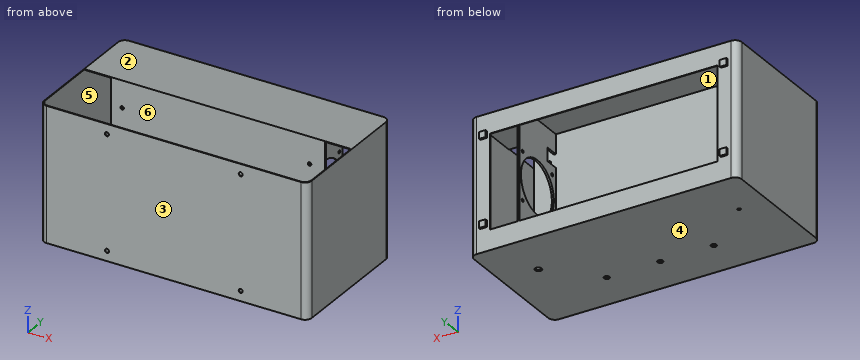
```python
from build123d import *

# Parameters (mm, degrees)
SKETCH1_W                 = 400
SKETCH1_H                 = 200
KHUNG_TRONG_DEPTH         = 100
SKETCH2_W                 = 398
SKETCH2_H                 = 198
DO_DAY_1MM_DEPTH          = 198
FILLET_10MM_4_GOC_R       = 10
SKETCH3_W                 = 320
SKETCH3_H                 = 3
TRAN_GIA_DEPTH            = 198
SKETCH5_W                 = 3
SKETCH5_H                 = 198
GIA_DO_QUAT_DEPTH         = 89
SKETCH6_R                 = 40
LO_DAT_QUAT_DEPTH         = 3
SKETCH7_R                 = 2.3
CO_DINH_QUAT_DEPTH        = 3
SKETCH9_W                 = 20
SKETCH9_H                 = 20
LO_THONG_CHO_DEN_DEPTH    = 3
SKETCH10_R                = 2.6
GIA_DO_DEN_DEPTH          = 3
DAY_NGUON_DEN_QUAT_REACH  = 491.085
SKETCH12_R                = 5
DAY_NGUON_DEN_REACH       = 491.085
SKETCH13_R                = 2.5
F_2_THANH_RAY_TANG1_REACH = 459.822
SKETCH14_R                = 3
GAN_CAM_BIEN_REACH        = 491.085
SKETCH15_R                = 4.1
SKETCH16_W                = 340
SKETCH16_H                = 140
NAP_THAM_DEPTH            = 1
SKETCH18_W                = 399
SKETCH18_H                = 1
CHE_TRAN_DEPTH            = 93
FILLET4_R                 = 10
SKETCH19_W                = 10
SKETCH19_H                = 10
CHOT_CO_DINH_DEPTH        = 3


with BuildPart() as part:
    # Sketch1 → khung_trong (new, symmetric)
    with BuildSketch(Plane.XY):
        with Locations((200, 100)):
            Rectangle(SKETCH1_W, SKETCH1_H)
    extrude(amount=KHUNG_TRONG_DEPTH, both=True)

    # Sketch2 → do_day_1mm (cut)
    with BuildSketch(Plane.XY.offset(100)):
        with Locations((200, 100)):
            Rectangle(SKETCH2_W, SKETCH2_H)
    extrude(amount=-DO_DAY_1MM_DEPTH, mode=Mode.SUBTRACT)

    # Fillet_10mm_4_goc
    fillet_10mm_4_goc_edges = [part.edges().sort_by_distance(p)[0] for p in [
        (1, 1, 1),
        (1, 199, 1),
        (399, 199, 1),
        (399, 1, 1),
        (0, 200, 0),
        (400, 200, 0),
        (400, 0, 0),
        (0, 0, 0),
    ]]
    fillet(fillet_10mm_4_goc_edges, radius=FILLET_10MM_4_GOC_R)

    # Sketch3 → tran_gia (add)
    with BuildSketch(Plane.XY.offset(-98)):
        with Locations((200, 108.5)):
            Rectangle(SKETCH3_W, SKETCH3_H)
    extrude(amount=TRAN_GIA_DEPTH)

    # Sketch5 → gia_do_quat (add)
    with BuildSketch(Plane(origin=(0, 110, 0), x_dir=(1, 0, 0), z_dir=(0, 1, 0))):
        with Locations((328.5, -1)):
            Rectangle(SKETCH5_W, SKETCH5_H)
    extrude(amount=GIA_DO_QUAT_DEPTH)

    # Sketch6 → lo_dat_quat (cut)
    with BuildSketch(Plane.ZY.offset(-327)):
        with Locations((0, 155)):
            Circle(SKETCH6_R)
    extrude(amount=-LO_DAT_QUAT_DEPTH, mode=Mode.SUBTRACT)

    # Sketch7 → co_dinh_quat (cut)
    with BuildSketch(Plane.ZY.offset(-327)):
        with Locations((-35.75, 190.75)):
            Circle(SKETCH7_R)
        with Locations((35.75, 190.75)):
            Circle(SKETCH7_R)
        with Locations((35.75, 119.25)):
            Circle(SKETCH7_R)
        with Locations((-35.75, 119.25)):
            Circle(SKETCH7_R)
    extrude(amount=-CO_DINH_QUAT_DEPTH, mode=Mode.SUBTRACT)

    # Sketch9 → lo_thong_cho _den (cut)
    with BuildSketch(Plane.ZY.offset(-327)):
        with Locations((-58, 120)):
            Rectangle(SKETCH9_W, SKETCH9_H)
        with Locations((60, 120)):
            Rectangle(SKETCH9_W, SKETCH9_H)
    extrude(amount=-LO_THONG_CHO_DEN_DEPTH, mode=Mode.SUBTRACT)

    # Sketch10 → gia_do_den (cut)
    with BuildSketch(Plane(origin=(0, 110, 0), x_dir=(1, 0, 0), z_dir=(0, 1, 0))):
        with Locations(Location((337, 58, 0), (0, 0, 270))):
            Circle(SKETCH10_R)
        with Locations(Location((337, -60, 0), (0, 0, 270))):
            Circle(SKETCH10_R)
        with Locations(Location((57, 58, 0), (0, 0, 270))):
            Circle(SKETCH10_R)
        with Locations(Location((57, -60, 0), (0, 0, 270))):
            Circle(SKETCH10_R)
    extrude(amount=-GIA_DO_DEN_DEPTH, mode=Mode.SUBTRACT)

    # Sketch12 → day_nguon_den_quat (cut, up to next)
    with BuildSketch(Plane.XY.offset(-98), mode=Mode.PRIVATE) as day_nguon_den_quat_sk1:
        with Locations((344, 125)):
            Circle(SKETCH12_R)
    day_nguon_den_quat_tool1 = extrude(day_nguon_den_quat_sk1.sketch, amount=-DAY_NGUON_DEN_QUAT_REACH, mode=Mode.PRIVATE) & part.part
    add(day_nguon_den_quat_tool1.solids().sort_by_distance((344, 125, -98))[0], mode=Mode.SUBTRACT)

    # Sketch13 → day_nguon_den (cut, up to next)
    with BuildSketch(Plane.XY.offset(-98), mode=Mode.PRIVATE) as day_nguon_den_sk1:
        with Locations((44, 125)):
            Circle(SKETCH13_R)
    day_nguon_den_tool1 = extrude(day_nguon_den_sk1.sketch, amount=-DAY_NGUON_DEN_REACH, mode=Mode.PRIVATE) & part.part
    add(day_nguon_den_tool1.solids().sort_by_distance((44, 125, -98))[0], mode=Mode.SUBTRACT)

    # Sketch14 → 2_thanh_ray_tang1 (cut, up to next)
    with BuildSketch(Plane(origin=(0, 1, 0), x_dir=(1, 0, 0), z_dir=(0, 1, 0)), mode=Mode.PRIVATE) as f_2_thanh_ray_tang1_sk1:
        with Locations(Location((100, 85, 0), (0, 0, 270))):
            Circle(SKETCH14_R)
    f_2_thanh_ray_tang1_tool1 = extrude(f_2_thanh_ray_tang1_sk1.sketch, amount=-F_2_THANH_RAY_TANG1_REACH, mode=Mode.PRIVATE) & part.part
    # Sketch14 → 2_thanh_ray_tang1 (cut, up to next)
    with BuildSketch(Plane(origin=(0, 1, 0), x_dir=(1, 0, 0), z_dir=(0, 1, 0)), mode=Mode.PRIVATE) as f_2_thanh_ray_tang1_sk2:
        with Locations(Location((300, 85, 0), (0, 0, 270))):
            Circle(SKETCH14_R)
    f_2_thanh_ray_tang1_tool2 = extrude(f_2_thanh_ray_tang1_sk2.sketch, amount=-F_2_THANH_RAY_TANG1_REACH, mode=Mode.PRIVATE) & part.part
    # Sketch14 → 2_thanh_ray_tang1 (cut, up to next)
    with BuildSketch(Plane(origin=(0, 1, 0), x_dir=(1, 0, 0), z_dir=(0, 1, 0)), mode=Mode.PRIVATE) as f_2_thanh_ray_tang1_sk3:
        with Locations(Location((300, -85, 0), (0, 0, 270))):
            Circle(SKETCH14_R)
    f_2_thanh_ray_tang1_tool3 = extrude(f_2_thanh_ray_tang1_sk3.sketch, amount=-F_2_THANH_RAY_TANG1_REACH, mode=Mode.PRIVATE) & part.part
    # Sketch14 → 2_thanh_ray_tang1 (cut, up to next)
    with BuildSketch(Plane(origin=(0, 1, 0), x_dir=(1, 0, 0), z_dir=(0, 1, 0)), mode=Mode.PRIVATE) as f_2_thanh_ray_tang1_sk4:
        with Locations(Location((100, -85, 0), (0, 0, 270))):
            Circle(SKETCH14_R)
    f_2_thanh_ray_tang1_tool4 = extrude(f_2_thanh_ray_tang1_sk4.sketch, amount=-F_2_THANH_RAY_TANG1_REACH, mode=Mode.PRIVATE) & part.part
    add(f_2_thanh_ray_tang1_tool1.solids().sort_by_distance((100, 1, -85))[0], mode=Mode.SUBTRACT)
    add(f_2_thanh_ray_tang1_tool2.solids().sort_by_distance((300, 1, -85))[0], mode=Mode.SUBTRACT)
    add(f_2_thanh_ray_tang1_tool3.solids().sort_by_distance((300, 1, 85))[0], mode=Mode.SUBTRACT)
    add(f_2_thanh_ray_tang1_tool4.solids().sort_by_distance((100, 1, 85))[0], mode=Mode.SUBTRACT)

    # Sketch15 → gan_cam_bien (cut, up to next)
    with BuildSketch(Plane.XY.offset(-98), mode=Mode.PRIVATE) as gan_cam_bien_sk1:
        with Locations((121, 61)):
            Circle(SKETCH15_R)
    gan_cam_bien_tool1 = extrude(gan_cam_bien_sk1.sketch, amount=-GAN_CAM_BIEN_REACH, mode=Mode.PRIVATE) & part.part
    # Sketch15 → gan_cam_bien (cut, up to next)
    with BuildSketch(Plane.XY.offset(-98), mode=Mode.PRIVATE) as gan_cam_bien_sk2:
        with Locations((201, 61)):
            Circle(SKETCH15_R)
    gan_cam_bien_tool2 = extrude(gan_cam_bien_sk2.sketch, amount=-GAN_CAM_BIEN_REACH, mode=Mode.PRIVATE) & part.part
    # Sketch15 → gan_cam_bien (cut, up to next)
    with BuildSketch(Plane.XY.offset(-98), mode=Mode.PRIVATE) as gan_cam_bien_sk3:
        with Locations((281, 61)):
            Circle(SKETCH15_R)
    gan_cam_bien_tool3 = extrude(gan_cam_bien_sk3.sketch, amount=-GAN_CAM_BIEN_REACH, mode=Mode.PRIVATE) & part.part
    add(gan_cam_bien_tool1.solids().sort_by_distance((121, 61, -98))[0], mode=Mode.SUBTRACT)
    add(gan_cam_bien_tool2.solids().sort_by_distance((201, 61, -98))[0], mode=Mode.SUBTRACT)
    add(gan_cam_bien_tool3.solids().sort_by_distance((281, 61, -98))[0], mode=Mode.SUBTRACT)

    # Sketch16 → nap_tham (cut)
    with BuildSketch(Plane(origin=(0, 200, 0), x_dir=(1, 0, 0), z_dir=(0, 1, 0))):
        with Locations((200, 0)):
            Rectangle(SKETCH16_W, SKETCH16_H)
    extrude(amount=-NAP_THAM_DEPTH, mode=Mode.SUBTRACT)

    # Sketch18 → che_tran (add)
    with BuildSketch(Plane.XZ.offset(-107)):
        with Locations((200.5, 99.5)):
            Rectangle(SKETCH18_W, SKETCH18_H)
    extrude(amount=-CHE_TRAN_DEPTH)

    # Fillet4
    # the kernel refuses this fillet: 10 mm, written as the material it takes off along each edge
    with BuildSketch(Plane(origin=(400, 200, 125), x_dir=(-1, 0, 0), z_dir=(0, 0, -1))) as fillet4_piece_1:
        with BuildLine():
            CenterArc((FILLET4_R, -FILLET4_R), FILLET4_R, 90, 90)
            Line((0, -FILLET4_R), (-FILLET4_R * 0.02, -FILLET4_R))
            Line((-FILLET4_R * 0.02, -FILLET4_R), (-FILLET4_R * 0.02, FILLET4_R * 0.02))
            Line((-FILLET4_R * 0.02, FILLET4_R * 0.02), (FILLET4_R, FILLET4_R * 0.02))
            Line((FILLET4_R, FILLET4_R * 0.02), (FILLET4_R, 0))
        make_face()
    extrude(amount=51, mode=Mode.SUBTRACT)
    with BuildSketch(Plane(origin=(1, 200, 76.5), x_dir=(1, 0, 0), z_dir=(0, 0, 1))) as fillet4_piece_2:
        with BuildLine():
            CenterArc((9, -10), FILLET4_R, 90, 64.158067237)
            Line((0, -5.641101056), (-0.18, -5.553923078))
            ThreePointArc((-0.18, -5.553923078), (-0.2, -2.820550528), (-0.2, 0))
            Line((-0.2, 0), (0, 0.2))
            Line((0, 0.2), (9, 0.2))
            Line((9, 0.2), (9, 0))
        make_face()
    extrude(amount=46, mode=Mode.SUBTRACT)

    # Sketch19 → chot_co_dinh (add)
    with BuildSketch(Plane(origin=(0, 200, 0), x_dir=(1, 0, 0), z_dir=(0, 1, 0))):
        with Locations((20, 60)):
            Rectangle(SKETCH19_W, SKETCH19_H)
        with Locations((380, 60)):
            Rectangle(SKETCH19_W, SKETCH19_H)
        with Locations((380, -70)):
            Rectangle(SKETCH19_W, SKETCH19_H)
        with Locations((20, -70)):
            Rectangle(SKETCH19_W, SKETCH19_H)
    extrude(amount=CHOT_CO_DINH_DEPTH)


solid = part.part
```
Geometry check sheet. Reference: the model listing, model coordinates, mm. Face numbers are marked on the shaded views. A direction names the side the tool comes from. Give positions to 0.01 mm unless a question says otherwise; leave off trailing zeros. Order: outer loops, then holes, each group sorted by start corner. A loop starts at its lowest first (then second) coordinate and runs counter-clockwise, first axis right, second up.
1. Gauge pin test, flat ends, axial feed: pin 1 Ø6 at (x, y) = (44, 125) entering from -Z; pin 2 Ø6.5 at (x, y) = (121, 61) entering from +Z; pin 3 Ø9.5 at (x, y) = (281, 61) entering from +Z; pin 4 Ø10 at (x, z) = (330.5, -0.5) entering from +Y. Record the tip position at first contact, or that the pin passes through.
2. Section check C-C, the plane y = 34.5. Enter the section's corners in (x, z).
3. Thickness scan on L1, parallel to Y at x = 359, z = 75.5; L2, parallel to X at y = 171, z = 46; L3, parallel to Z at x = 337, y = 109. Record the ranges inside material, lowest first.
4. Section check A-A, the plane x = 281. Enter the section's corners in (y, z), and give its area (3 significant figures).
5. Access from +Z, -Z, +X, -X, +Y, -Y to the whole of each face (thin tool, end or side, straight path). Record for the marked faces 4, 5 and 6.
6. Section check B-B, the plane z = 0. Give the number of separate pieces and of enclosed holes in the cut face, and give its area (3 significant figures).
7. Section check D-D, the plane x = 356. Enter the section's corners in (y, z), and give its area (3 significant figures).
8. Release check for a two-part mould opening along Z. For the marked faces 1, 2 and 3 record: pulls with the +Z half, pulls with the -Z half, needs draft (parallel to the pull), parting line crosses it, or undercut.
Values follow:
1. pin 1: stops at z = -100
1. pin 2: passes through
1. pin 3: stops at z = -98
1. pin 4: stops at y = 199
2. outline: (0, -100) - (400, -100) - (400, 100) - (399, 100) - (399, -98) - (1, -98) - (1, 100) - (0, 100) - close
3. L1: y = 0 to 1, 107 to 110, 199 to 200
3. L2: x = 0 to 1, 327 to 330, 399 to 400
3. L3: z = -100 to -60.6, -55.4 to 57.4, 62.6 to 100
4. outline: (0, -100) - (56.9, -100) - (56.9, -98) - (1, -98) - (1, 100) - (0, 100) - close; (65.1, -100) - (200, -100) - (200, -70) - (199, -70) - (199, -98) - (110, -98) - (110, 99) - (199, 99) - (199, 70) - (200, 70) - (200, 100) - (107, 100) - (107, -98) - (65.1, -98) - close
4. area: 1,320 mm2
5. face 4: -Z, +X, -X, +Y, -Y
5. face 5: none
5. face 6: +Z
6. separate pieces: 3
6. enclosed holes: 0
6. area: 1,840 mm2
7. outline: (0, -100) - (200, -100) - (200, -70) - (199, -70) - (199, -98) - (110, -98) - (110, 99) - (199, 99) - (199, 70) - (200, 70) - (200, 100) - (107, 100) - (107, -98) - (1, -98) - (1, 100) - (0, 100) - close
7. area: 1,340 mm2
8. face 1: undercut
8. face 2: pulls with the +Z half
8. face 3: needs draft
